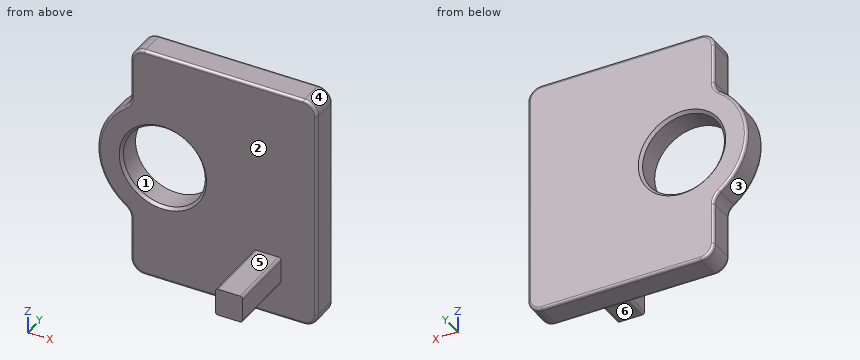
```python
from build123d import *

# Parameters (mm, degrees)
F0_R     = 15
F1_DEPTH = 10
F2_R     = 5
F3_SIZE  = 1
F4_R     = 1
F5_W     = 10
F5_H     = 10
F6_DEPTH = 25.4
F7_R     = 1


with BuildPart() as f1:
    # F0 (on Front) → F1 (new body)
    with BuildSketch(Plane.XZ):
        with BuildLine():
            Line((32.266531, 50.35542), (-35.933132, 50.35542))
            Line((-35.933132, 50.35542), (-35.933132, 28.043626))
            ThreePointArc((-35.933132, 28.043626), (-48.068501, 7.269355), (-35.933132, -13.504916))
            Line((-35.933132, -13.504916), (-35.933132, -36.456365))
            Line((-35.933132, -36.456365), (32.266531, -36.456365))
            Line((32.266531, -36.456365), (32.266531, 50.35542))
        make_face()
        with Locations((-24.219309, 7.269355)):
            Circle(F0_R, mode=Mode.SUBTRACT)
    extrude(amount=-F1_DEPTH)

    # F2
    f2_edges = [f1.edges().sort_by_distance(p)[0] for p in [
        (-35.933132, 5, 28.043626),
        (-35.933132, 5, -13.504916),
        (-35.933132, 5, 50.35542),
        (-35.933132, 5, -36.456365),
        (32.266531, 5, 50.35542),
        (32.266531, 5, -36.456365),
    ]]
    fillet(f2_edges, radius=F2_R)

    # F3
    f3_edges = [f1.edges().sort_by_distance(p)[0] for p in [
        (-39.219309, 10, 7.269355),
        (-39.219309, 0, 7.269355),
    ]]
    chamfer(f3_edges, length=F3_SIZE)

    # F4
    f4_edges = [f1.edges().sort_by_distance(p)[0] for p in [
        (-1.8333, 10, 50.35542),
        (32.266531, 0, 6.949527),
    ]]
    fillet(f4_edges, radius=F4_R)

    # F5 (on Front) → F6 (join)
    with BuildSketch(Plane.XZ):
        with Locations((14.072881, -18.364601)):
            Rectangle(F5_W, F5_H)
    extrude(amount=F6_DEPTH)

    # F7
    f7_edges = [f1.edges().sort_by_distance(p)[0] for p in [
        (19.072881, -12.7, -23.364601),
        (9.072881, -12.7, -23.364601),
        (9.072881, -12.7, -13.364601),
        (19.072881, -12.7, -13.364601),
    ]]
    fillet(f7_edges, radius=F7_R)


solid = f1.part
```
Input: part model. Units: mm. Frame: model coordinates. Face numbers are marked on the shaded views. A direction names the side the tool comes from. Coordinates: 2 decimals unless noted, no trailing zeros. Write each loop counter-clockwise with the first axis right and the second up, starting at its lowest first coordinate (ties: lowest second). Pieces come first, ordered by that corner, then holes. Notation, with made-up numbers: (55, -26) -> (113, -26) arc R24 cw to (113, -2) -> close; hole circle Ø1 at (25, 34.5). An arc over 180 degrees is marked (long way). Write each question's results on one line, items separated by ' | '.
Item 1: Section query A-A on y = -3.5. Return loops of the section in (x, z), plus the area to 3 significant figures.
Conclusion:
outline: (9.07, -22.36) arc R1 ccw to (10.07, -23.36) -> (18.07, -23.36) arc R1 ccw to (19.07, -22.36) -> (19.07, -14.36) arc R1 ccw to (18.07, -13.36) -> (10.07, -13.36) arc R1 ccw to (9.07, -14.36) -> close | area: 99.1 mm^2
Item 2: Section query B-B on z = -19. Return loops of the section in (x, y), plus the area to 3 significant figures.
Conclusion:
outline: (-35.93, 1) arc R1 ccw to (-34.93, 0) -> (9.07, 0) -> (9.07, -25.4) -> (19.07, -25.4) -> (19.07, 0) -> (31.27, 0) arc R1 ccw to (32.27, 1) -> (32.27, 9) arc R1 ccw to (31.27, 10) -> (-34.93, 10) arc R1 ccw to (-35.93, 9) -> close | area: 935 mm^2
Item 3: Section query D-D on x = 15. Return loops of the section in (y, z), plus the area to 3 significant figures.
Conclusion:
outline: (-25.4, -23.36) -> (0, -23.36) -> (0, -35.46) arc R1 ccw to (1, -36.46) -> (9, -36.46) arc R1 ccw to (10, -35.46) -> (10, 49.36) arc R1 ccw to (9, 50.36) -> (1, 50.36) arc R1 ccw to (0, 49.36) -> (0, -13.36) -> (-25.4, -13.36) -> close | area: 1,120 mm^2
Item 4: Material intervals for probe 1 along Y at (x, z) = (-19, -16); probe 2 along Z at (x, y) = (27.5, 7.5); probe 3 along X at (y, z) = (3, 6.5), sorted ascending.
Conclusion:
probe 1: y = 0 to 10 | probe 2: z = -36.45 to 50.35 | probe 3: x = -48.06 to -39.2, -9.24 to 32.27
Item 5: Mould query, pull axis X, two halves, no side actions, for the marked faces 1, 2 and 3. Classes: +X half, -X half, draft (parallel to the pull), parting line (faces both ways), or undercut.
Conclusion:
face 1: undercut | face 2: draft | face 3: -X half
Item 6: Set-up query: the marked faces 4, 5 and 6. Return all of +Z, -Z, +X, -X, +Y, -Y with unobstructed straight access to the full face (end or side cutting, diameter ignored); none if empty.
Conclusion:
face 4: +Z, +X, +Y, -Y | face 5: +Z, +X, -X, -Y | face 6: -Z, +X, -X, -Y
Item 7: Pin query (flat end, axial travel): pin 1 Ø10 at (y, z) = (-8, -19) entering from -X; pin 2 Ø3 at (x, z) = (-4, 33.5) entering from -Y; pin 3 Ø2.5 at (y, z) = (4.5, -23) entering from -X. Return the tip coordinate at first contact, or that it passes through.
Conclusion:
pin 1: stops at x = 9.07 | pin 2: stops at y = 0 | pin 3: stops at x = -35.93
Item 8: Section query C-C on x = 4. Return loops of the section in (y, z).
Conclusion:
outline: (0, -35.46) arc R1 ccw to (1, -36.46) -> (9, -36.46) arc R1 ccw to (10, -35.46) -> (10, 49.36) arc R1 ccw to (9, 50.36) -> (1, 50.36) arc R1 ccw to (0, 49.36) -> close
